The listing builds one solid part. Answer for the finished solid, in the listing's coordinates (mm). A direction names the side the tool comes from. Coordinates: 2 decimals unless noted, no trailing zeros. Loops run counter-clockwise (first coordinate to the right, second up) from the corner with the lowest first, then second, coordinate; pieces in that order, holes last. Notation, with made-up numbers: M 67.25,41.25 L 99.25,41.25 A12 cw 99.25,49.25 Z; hole C -10,83 d2. An arc over 180 degrees is marked long. Answer as CSV lines item,"result". Start each with the question number.
```python
from build123d import *

# Parameters (mm, degrees)
EXTRUDE1_DEPTH = 5.08
SHELL1_T       = -0.508
EXTRUDE2_REACH = 6.572
SKETCH2_W      = 1.27
SKETCH2_H      = 25.4508


with BuildPart() as part:
    # Sketch1 → Extrude1 (new body)
    with BuildSketch(Plane(origin=(0, 0, 0), x_dir=(1, 0, 0), z_dir=(0, 1, 0))):
        Polygon((12.7, 0), (-12.7, 0), (-7.9375, 19.05), (-7.9375, 25.4508), (7.9375, 25.4508), (7.9375, 19.05), align=None)
    extrude(amount=EXTRUDE1_DEPTH)

    # Shell1
    shell1_openings = [part.faces().sort_by_distance(p)[0] for p in [
        (0, 2.54, -25.4508),
        (0, 2.54, 0),
    ]]
    offset(amount=SHELL1_T, openings=shell1_openings, kind=Kind.INTERSECTION)

    # Sketch2 → Extrude2 (add, up to next)
    with BuildSketch(Plane(origin=(0, 0.508, 0), x_dir=(-1, 0, 0), z_dir=(0, 1, 0)), mode=Mode.PRIVATE) as extrude2_sk1:
        with Locations((0, -12.7254)):
            Rectangle(SKETCH2_W, SKETCH2_H)
    extrude2_tool1 = extrude(extrude2_sk1.sketch, amount=EXTRUDE2_REACH, mode=Mode.PRIVATE) - part.part
    add(extrude2_tool1.solids().sort_by_distance((0, 0.508, -12.7254))[0])


solid = part.part
```
Item 1: For faces 4 (the face through (-7.938, 3, -22)), 5 (the face through (9.77, 2.51, -9.63)), 6 (the face through (7.938, 3, -22)), 7 (the face through (-7.43, 3, -22)), determine the directions among +Z, -Z, +X, -X, +Y, -Y from which every point of the face is accessible in a straight line to the end or side of a thin tool.
Item 2: For a pull along X with two mould halves and no side action, classify faces 1 (the face through (0, 0, -10)), 2 (the face through (10.285, 2.504, -9.658)), 3 (the face through (0.635, 3, -13)) as pulls with the +X half, pulls with the -X half, needs draft (parallel to the pull), parting line crosses it, or undercut.
Item 3: Section B-B on z = -23.25 is taken. Determine the outline of the cut face in (x, y) (1 decimal).
Item 4: Consider line 1 (X direction, y = 4.35, z = -24) (1 decimal); line 2 (Y direction, x = -3.25, z = -1.5); line 3 (X direction, y = 3.15, z = -4) (3 decimals). Determine where each line is inside the solid, lowest interval first.
Item 5: Section A-A on x = 1.75 is taken. Determine the outline of the cut face in (y, z).
Item 6: Section D-D on z = -11.75 is taken. Determine the outline of the cut face in (x, y) (1 decimal), then the cut area to 3 significant figures.
Item 7: Each of these flat-tipped pins is pushed along its axis until it touches: P1, Ø1.2, axis at y = 3, z = -21.5, coming from the +X side; P2, Ø2.5, axis at y = 2.5, z = -23.5, coming from the -X side; P3, Ø1.2, axis at y = 3, z = -7, coming from the -X side. Where does it stop, or does it pass through?
Item 8: Section C-C on y = 1.1 is taken. State how many separate pieces and enclosed holes the cut face has, then the cut area to 3 significant figures.
Results are:
1,face 4,"-Z, -X, +Y, -Y"
1,face 5,"+Z"
1,face 6,"-Z, +X, +Y, -Y"
1,face 7,"+Z, -Z"
2,face 1,"needs draft"
2,face 2,"pulls with the +X half"
2,face 3,"undercut"
3,outline,"M -7.9,0 L 7.9,0 L 7.9,5.1 L -7.9,5.1 Z; hole M -7.4,0.5 L -0.6,0.5 L -0.6,4.6 L -7.4,4.6 Z; hole M 0.6,0.5 L 7.4,0.5 L 7.4,4.6 L 0.6,4.6 Z"
4,line 1,"-7.9 to -7.4, -0.6 to 0.6, 7.4 to 7.9"
4,line 2,"0 to 0.51, 4.57 to 5.08"
4,line 3,"-11.7 to -11.176, -0.635 to 0.635, 11.176 to 11.7"
5,outline,"M 0,-25.45 L 0.51,-25.45 L 0.51,0 L 0,0 Z; M 4.57,-25.45 L 5.08,-25.45 L 5.08,0 L 4.57,0 Z"
6,outline,"M -9.8,0 L 9.8,0 L 9.8,5.1 L -9.8,5.1 Z; hole M -9.2,0.5 L -0.6,0.5 L -0.6,4.6 L -9.2,4.6 Z; hole M 0.6,0.5 L 9.2,0.5 L 9.2,4.6 L 0.6,4.6 Z"
6,area,"29.3 mm²"
7,P1,"x = 7.94"
7,P2,"x = -7.94"
7,P3,"x = -11.1"
8,separate pieces,"3"
8,enclosed holes,"0"
8,area,"58.8 mm²"
